Work out the finished part from the listing and answer in its coordinate system (mm). A direction names the side the tool comes from. Coordinates: 2 decimals unless noted, no trailing zeros. Order: outer loops, then holes, each group sorted by start corner. A loop starts at its lowest first (then second) coordinate and runs counter-clockwise, first axis right, second up. Notation, with made-up numbers: M 65.25,45.25 L 100.25,45.25 A18 ccw 100.25,65.25 Z; hole C 76.25,31 d7. An arc over 180 degrees is marked long. Use a Markdown table: item, result.
from build123d import *

# Parameters (mm, degrees)
PAD_DEPTH    = 15
SKETCH001_R  = 2.5
POCKET_DEPTH = 10


with BuildPart() as part:
    # Sketch → Pad (new body)
    with BuildSketch(Plane.XY):
        with BuildLine():
            ThreePointArc((57, 0), (0, 57), (-57, 0))
            Line((-84.505814, 0), (-57, 0))
            Line((-84.505814, 8), (-84.505814, 0))
            Line((-64.505814, 8), (-84.505814, 8))
            ThreePointArc((64.505814, 8), (0, 65), (-64.505814, 8))
            Line((64.505814, 8), (84.505814, 8))
            Line((84.505814, 8), (84.505814, 0))
            Line((84.505814, 0), (57, 0))
        make_face()
    extrude(amount=PAD_DEPTH)

    # Sketch001 (on Face1 of Pad) → Pocket (cut)
    with BuildSketch(Plane(origin=(0, 8, 0), x_dir=(-1, 0, 0), z_dir=(0, 1, 0))):
        with Locations((-75, 7.5)):
            Circle(SKETCH001_R)
        with Locations((75, 7.5)):
            Circle(SKETCH001_R)
    extrude(amount=-POCKET_DEPTH, mode=Mode.SUBTRACT)


solid = part.part
(1) Straight lines are drawn through the part: L1, parallel to Z at x = -75, y = 3.5; L2, parallel to X at y = 9, z = 1; L3, parallel to X at y = 27.5, z = 7.75. For each, find the intervals that lie inside material, in ascending order.
Conclusion:
| item | result |
|---|---|
| L1 | 0 to 5, 10 to 15 |
| L2 | -64.37 to -56.28, 56.28 to 64.37 |
| L3 | -58.9 to -49.93, 49.93 to 58.9 |
(2) Which of the six approach directions +Z, -Z, +X, -X, +Y, -Y give full straight-line access (tool end or side, diameter ignored) to faces 1 (the flat face through (72, 8, 7)), 2 (the cylindrical face through (77, 4, 6)), 3 (the flat face through (-72, 8, 7))?
Conclusion:
| item | result |
|---|---|
| face 1 | +Z, -Z, +X, +Y |
| face 2 | +Y, -Y |
| face 3 | +Z, -Z, -X, +Y |
(3) A cutting plane is placed at B-B (x = 75). Determine the outline of the cut face in (y, z).
Conclusion:
| item | result |
|---|---|
| outline | M 0,0 L 8,0 L 8,5 L 0,5 Z; M 0,10 L 8,10 L 8,15 L 0,15 Z |
(4) Determine the mould class of faces 4 (the flat face through (84.506, 4, 7)), 5 (the cylindrical face through (-73, 4, 6)), 6 (the cylindrical face through (1.317, 64.987, 7.395)) for opening direction X: pulls with the +X half, pulls with the -X half, needs draft (parallel to the pull), parting line crosses it, or undercut.
Conclusion:
| item | result |
|---|---|
| face 4 | pulls with the +X half |
| face 5 | undercut |
| face 6 | parting line crosses it |
(5) A cutting plane is placed at A-A (z = 7.5). Determine the outline of the cut face in (x, y), then the cut area to 3 significant figures.
Conclusion:
| item | result |
|---|---|
| outline | M -84.51,0 L -77.5,0 L -77.5,8 L -84.51,8 Z; M -72.5,0 L -57,0 A57 cw 57,0 L 72.5,0 L 72.5,8 L 64.51,8 A65 ccw -64.51,8 L -72.5,8 Z; M 77.5,0 L 84.51,0 L 84.51,8 L 77.5,8 Z |
| area | 1,770 mm2 |
(6) A cutting plane is placed at C-C (y = 25). Determine the outline of the cut face in (x, z) (3 decimals).
Conclusion:
| item | result |
|---|---|
| outline | M -60,0 L -51.225,0 L -51.225,15 L -60,15 Z; M 51.225,0 L 60,0 L 60,15 L 51.225,15 Z |
(7) A cutting plane is placed at D-D (x = 21). Determine the outline of the cut face in (y, z).
Conclusion:
| item | result |
|---|---|
| outline | M 52.99,0 L 61.51,0 L 61.51,15 L 52.99,15 Z |
(8) Given P1, Ø6.5, axis at x = -75, z = 7.5, coming from the +Y side; P2, Ø5, axis at x = 61.5, z = 2, coming from the +Y side; P3, Ø8, axis at y = 31, z = 7, coming from the -X side, each flat-ended and moving along its own axis, determine where each tip first touches the part or whether it passes through.
Conclusion:
| item | result |
|---|---|
| P1 | y = 8 |
| P2 | y = 27.28 |
| P3 | x = -59.13 |
